```python
from build123d import *

# Parameters (mm, degrees)
BOSS_EXTRUDE1_DEPTH = 19.05
SKETCH2_R           = 2.9845
BOSS_EXTRUDE2_DEPTH = 48.895
FILLET1_R           = 0.381
FILLET2_R           = 0.381
FILLET3_R           = 0.508
FILLET4_R           = 0.508


with BuildPart() as part:
    # Sketch1 → Boss-Extrude1 (new body)
    with BuildSketch(Plane.XY):
        Polygon((2.410509543, -4.175125), (4.821019085, 0), (2.410509543, 4.175125), (-2.410509543, 4.175125), (-4.821019085, 0), (-2.410509543, -4.175125), align=None)
    extrude(amount=BOSS_EXTRUDE1_DEPTH)

    # Sketch2 → Boss-Extrude2 (add)
    with BuildSketch(Plane.XY.offset(19.05)):
        Circle(SKETCH2_R)
    extrude(amount=BOSS_EXTRUDE2_DEPTH)

    # Fillet1
    fillet1_edges = [part.edges().sort_by_distance(p)[0] for p in [
        (-2.9845, 0, 67.945),
    ]]
    fillet(fillet1_edges, radius=FILLET1_R)

    # Fillet2
    fillet2_edges = [part.edges().sort_by_distance(p)[0] for p in [
        (-2.9845, 0, 19.05),
    ]]
    fillet(fillet2_edges, radius=FILLET2_R)

    # Fillet3
    fillet3_edges = [part.edges().sort_by_distance(p)[0] for p in [
        (3.615764314, 2.0875625, 19.05),
        (0, 4.175125, 19.05),
        (-3.615764314, 2.0875625, 19.05),
        (-3.615764314, -2.0875625, 19.05),
        (0, -4.175125, 19.05),
        (-3.615764314, -2.0875625, 0),
        (-3.615764314, 2.0875625, 0),
        (0, 4.175125, 0),
        (3.615764314, 2.0875625, 0),
        (3.615764314, -2.0875625, 0),
        (0, -4.175125, 0),
        (3.615764314, -2.0875625, 19.05),
    ]]
    fillet(fillet3_edges, radius=FILLET3_R)

    # Fillet4
    fillet4_edges = [part.edges().sort_by_distance(p)[0] for p in [
        (4.821019085, 0, 9.525),
        (2.410509543, -4.175125, 9.525),
        (2.410509543, 4.175125, 9.525),
        (-2.410509543, -4.175125, 9.525),
        (-2.410509543, 4.175125, 9.525),
        (-4.821019085, 0, 9.525),
        (-4.634149245, 0, 0.136202851),
        (-2.317074623, 4.013290972, 0.136202851),
        (-2.317074623, -4.013290972, 0.136202851),
        (2.317074623, 4.013290972, 0.136202851),
        (2.317074623, -4.013290972, 0.136202851),
        (4.634149245, 0, 0.136202851),
        (-2.317074623, -4.013290972, 18.913797149),
        (-4.634149245, 0, 18.913797149),
        (2.317074623, -4.013290972, 18.913797149),
        (-2.317074623, 4.013290972, 18.913797149),
        (4.634149245, 0, 18.913797149),
        (2.317074623, 4.013290972, 18.913797149),
    ]]
    fillet(fillet4_edges, radius=FILLET4_R)


solid = part.part
```
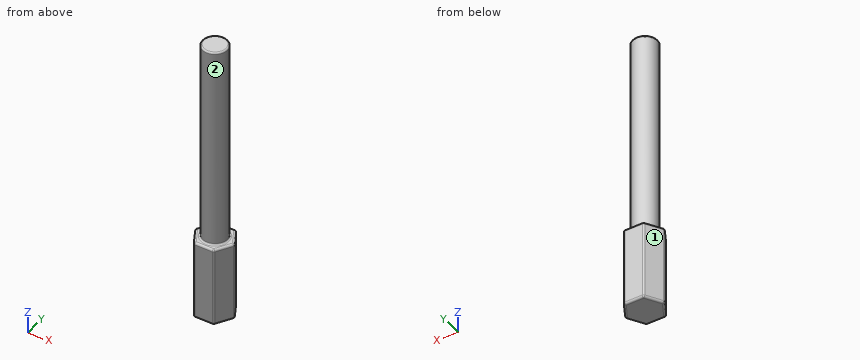
Geometry check sheet. Reference: the model listing, model coordinates, mm. Face numbers are marked on the shaded views. A direction names the side the tool comes from. Coordinates: 2 decimals unless noted, no trailing zeros. Write each loop counter-clockwise with the first axis right and the second up, starting at its lowest first coordinate (ties: lowest second). Pieces come first, ordered by that corner, then holes. Notation, with made-up numbers: M 43,82.5 L 83,82.5 A27 cw 83,121.5 Z; hole C 46.5,42.5 d2. An arc over 180 degrees is marked long. One line per item, written item: value. Start each with the question number.
(1) Depth check by flat-ended pin: pin 1 (4 mm diameter, centred on x = 1, y = 0, fed in from -Z); pin 2 (1.5 mm diameter, centred on x = 0.5, z = 34.5, fed in from -Y); pin 3 (3 mm diameter, centred on y = -1.5, z = 46.5, fed in from -X); pin 4 (1.5 mm diameter, centred on y = -2.5, z = 23.5, fed in from +X). Enter the tip coordinate at first touch or a pass-through.
(2) Sectioned sample at C-C, the plane z = 49. Enter the section's corners in (x, y), and give its area (3 significant figures).
(3) Sectioned sample at A-A, the plane z = 12. Enter the section's corners in (x, y).
(4) Tool access check on the marked faces 1 and 2. Record the directions out of +Z, -Z, +X, -X, +Y, -Y that give a thin tool (end or side, any length) a straight path to the whole face; none if there is none.
(5) Scan lines: line 1 along X through (y, z) = (-2.5, 16); line 2 along Z through (x, y) = (-1.75, 3.75); line 3 along X through (y, z) = (0.25, 23.5). Record each from-to range of solid material in increasing order. Write a range as [from, to].
Filled sheet:
1. pin 1: z = 0
1. pin 2: y = -2.98
1. pin 3: x = -2.98
1. pin 4: x = 2.42
2. outline: C 0,0 d5.97
2. area: 28.0 mm²
3. outline: M -4.67,-0.25 L -2.56,-3.92 A0.51 ccw -2.12,-4.18 L 2.12,-4.18 A0.51 ccw 2.56,-3.92 L 4.67,-0.25 A0.51 ccw 4.67,0.25 L 2.56,3.92 A0.51 ccw 2.12,4.18 L -2.12,4.18 A0.51 ccw -2.56,3.92 L -4.67,0.25 A0.51 ccw Z
4. face 1: +Z, -Z, -X, +Y
4. face 2: +Z
5. line 1: [-3.38, 3.38]
5. line 2: [0.01, 19.04]
5. line 3: [-2.97, 2.97]
